Read the model definition and answer for the solid it produces. Units are mm, in the model's axes. A direction names the side the tool comes from. Give positions to 0.01 mm unless a question says otherwise; leave off trailing zeros. Write each loop counter-clockwise with the first axis right and the second up, starting at its lowest first coordinate (ties: lowest second). Pieces come first, ordered by that corner, then holes. Notation, with made-up numbers: (-20.75, 88) -> (17.25, 88) arc R15 ccw to (17.25, 96) -> close; hole circle Ø7 at (76.25, 75.5). An arc over 180 degrees is marked (long way). Write item = value, one per line.
from build123d import *

# Parameters (mm, degrees)
SKETCH1_W                = 120
SKETCH1_H                = 82
BOSS_EXTRUDE1_DEPTH      = 10
BOSS_EXTRUDE4_DEPTH      = 82
FILLET2_R                = 20
BOSS_EXTRUDE5_DEPTH      = 100
M6_CLEARANCE_HOLE1_D     = 6.6
M6_CLEARANCE_HOLE1_DEPTH = 10


with BuildPart() as part:
    # Sketch1 → Boss-Extrude1 (new body)
    with BuildSketch(Plane(origin=(0, 0, 0), x_dir=(0, 0, -1), z_dir=(1, 0, 0))):
        Rectangle(SKETCH1_W, SKETCH1_H)
    extrude(amount=BOSS_EXTRUDE1_DEPTH)

    # Sketch6 → Boss-Extrude4 (add)
    with BuildSketch(Plane(origin=(0, 41, 0), x_dir=(1, 0, 0), z_dir=(0, 1, 0))):
        Polygon((0, 60), (0, 70), (10, 60), align=None)
        Polygon((0, -60), (0, -70), (10, -60), align=None)
    extrude(amount=-BOSS_EXTRUDE4_DEPTH)

    # Fillet2
    fillet2_edges = [part.edges().sort_by_distance(p)[0] for p in [
        (10, 0, 60),
        (10, 0, -60),
    ]]
    fillet(fillet2_edges, radius=FILLET2_R)

    # Sketch7 → Boss-Extrude5 (add)
    with BuildSketch(Plane(origin=(10, 0, 0), x_dir=(0, 0, -1), z_dir=(1, 0, 0))):
        with BuildLine():
            Line((-22.18, -32.18), (22.18, -32.18))
            ThreePointArc((22.18, -32.18), (29.251067812, -29.251067812), (32.18, -22.18))
            Line((32.18, -22.18), (32.18, 22.18))
            ThreePointArc((32.18, 22.18), (29.251067812, 29.251067812), (22.18, 32.18))
            Line((22.18, 32.18), (-22.18, 32.18))
            ThreePointArc((-22.18, 32.18), (-29.251067812, 29.251067812), (-32.18, 22.18))
            Line((-32.18, 22.18), (-32.18, -22.18))
            ThreePointArc((-32.18, -22.18), (-29.251067812, -29.251067812), (-22.18, -32.18))
        make_face()
        with BuildLine():
            Line((-17.18, -27.18), (17.18, -27.18))
            ThreePointArc((17.18, -27.18), (24.251067812, -24.251067812), (27.18, -17.18))
            Line((27.18, -17.18), (27.18, 17.18))
            ThreePointArc((27.18, 17.18), (24.251067812, 24.251067812), (17.18, 27.18))
            Line((17.18, 27.18), (-17.18, 27.18))
            ThreePointArc((-17.18, 27.18), (-24.251067812, 24.251067812), (-27.18, 17.18))
            Line((-27.18, 17.18), (-27.18, -17.18))
            ThreePointArc((-27.18, -17.18), (-24.251067812, -24.251067812), (-17.18, -27.18))
        make_face(mode=Mode.SUBTRACT)
    extrude(amount=BOSS_EXTRUDE5_DEPTH)

    # M6 Clearance Hole1
    with Locations(Plane(origin=(10, 0, 0), x_dir=(0, 0, -1), z_dir=(1, 0, 0))):
        with Locations((-40, 33.5), (40, 33.5), (40, -33.5), (-40, -33.5)):
            Hole(M6_CLEARANCE_HOLE1_D / 2, depth=M6_CLEARANCE_HOLE1_DEPTH)


solid = part.part
(1) For a pull along Y with two mould halves and no side action, classify faces 6 (the cylindrical face through (59.3, -29.2, 29.3)), 7 (the flat face through (110, 0, -28)), 8 (the cylindrical face through (59.3, 24.3, 24.2)) as released by +Y, released by -Y, zero draft, split by the parting line, or undercut.
Checks:
face_6 = released by -Y
face_7 = zero draft
face_8 = undercut
(2) The part is cut by section D-D on z = 7. Determine the outline of the cut face in (x, y).
Checks:
outline = (0, -41) -> (10, -41) -> (10, -32.18) -> (110, -32.18) -> (110, -27.18) -> (10, -27.18) -> (10, 27.18) -> (110, 27.18) -> (110, 32.18) -> (10, 32.18) -> (10, 41) -> (0, 41) -> close
(3) Consider L1, parallel to Y at x = 3, z = 40; L2, parallel to Z at x = 27.5, y = -7; L3, parallel to Z at x = 4, y = -33. Determine where each line is inside the solid, lowest interval first.
Checks:
L1 = -41 to -36.8, -30.2 to 30.2, 36.8 to 41
L2 = -32.18 to -27.18, 27.18 to 32.18
L3 = -66 to -43.26, -36.74 to 36.74, 43.26 to 66
(4) The part is cut by section C-C on y = -8. Determine the outline of the cut face in (x, z), plus the area to 3 significant figures.
Checks:
outline = (0, -70) -> (4.14, -65.86) arc R20 ccw to (10, -51.72) -> (10, -32.18) -> (110, -32.18) -> (110, -27.18) -> (10, -27.18) -> (10, 27.18) -> (110, 27.18) -> (110, 32.18) -> (10, 32.18) -> (10, 51.72) arc R20 ccw to (4.14, 65.86) -> (0, 70) -> close
area = 2,280 mm²
(5) The part is cut by section B-B on x = 68.5. Determine the outline of the cut face in (y, z), plus the area to 3 significant figures.
Checks:
outline = (-32.18, -22.18) arc R10 ccw to (-22.18, -32.18) -> (22.18, -32.18) arc R10 ccw to (32.18, -22.18) -> (32.18, 22.18) arc R10 ccw to (22.18, 32.18) -> (-22.18, 32.18) arc R10 ccw to (-32.18, 22.18) -> close; hole (-27.18, -17.18) arc R10 ccw to (-17.18, -27.18) -> (17.18, -27.18) arc R10 ccw to (27.18, -17.18) -> (27.18, 17.18) arc R10 ccw to (17.18, 27.18) -> (-17.18, 27.18) arc R10 ccw to (-27.18, 17.18) -> close
area = 1,190 mm²
(6) The part is cut by section A-A on z = -40. Determine the outline of the cut face in (x, y), plus the area to 3 significant figures.
Checks:
outline = (0, -41) -> (10, -41) -> (10, -36.8) -> (0, -36.8) -> close; (0, -30.2) -> (10, -30.2) -> (10, 30.2) -> (0, 30.2) -> close; (0, 36.8) -> (10, 36.8) -> (10, 41) -> (0, 41) -> close
area = 688 mm²
(7) A tool of negligible diameter and unlimited length cuts with its end or side. For faces 1 (the cylindrical face through (59.3, -29.3, -29.2)), 2 (the flat face through (59, 32.18, 0)), 3 (the flat face through (59, 0, -27.18)), 4 (the flat face through (59, 0, -32.18)), 5 (the flat face through (59, 0, 32.18)), from which of +Z, -Z, +X, -X, +Y, -Y can it reach the whole face along a straight path? Write none if from no direction.
Checks:
face_1 = -Z, +X, -Y
face_2 = +Z, -Z, +X, +Y
face_3 = +X
face_4 = -Z, +X, +Y, -Y
face_5 = +Z, +X, +Y, -Y
(8) Given P1, Ø22, axis at x = 53.5, y = -2.5, coming from the -Z side; P2, Ø2, axis at x = 72.5, z = -21.5, coming from the +Y side; P3, Ø13.5, axis at x = 37.5, y = -1, coming from the +Z side; P4, Ø6, axis at y = -33.5, z = 40, coming from the -X side, each flat-ended and moving along its own axis, determine where each tip first touches the part or whether it passes through.
Checks:
P1 = -32.18
P2 = 32.18
P3 = 32.18
P4 = through
